Input: part model. Units: mm. Frame: model coordinates. A direction names the side the tool comes from. Coordinates: 2 decimals unless noted, no trailing zeros. Write each loop counter-clockwise with the first axis right and the second up, starting at its lowest first coordinate (ties: lowest second). Pieces come first, ordered by that corner, then holes. Notation, with made-up numbers: M 53,-37.5 L 92,-37.5 A36 cw 92,-0.5 Z; hole C 46.25,86.5 d7. An arc over 180 degrees is marked long. Use one line per item in the form item = value.
from build123d import *

# Parameters (mm, degrees)
F0_W     = 200.66
F0_H     = 63.5
F1_DEPTH = 63.5
F2_W     = 200.66
F2_H     = 12.954
F2_W_2   = 175.26
F3_DEPTH = 3.1242


with BuildPart() as f1:
    # F0 (on Top) → F1 (new body)
    with BuildSketch(Plane.XY):
        with Locations((-100.33, 31.75)):
            Rectangle(F0_W, F0_H)
    extrude(amount=-F1_DEPTH)

    # F2 (on face) → F3 (cut)
    with BuildSketch(Plane.XY):
        with Locations((-100.33, 6.477)):
            Rectangle(F2_W, F2_H)
        with Locations((-87.63, 57.023)):
            Rectangle(F2_W_2, F2_H)
    extrude(amount=-F3_DEPTH, mode=Mode.SUBTRACT)


solid = f1.part
(1) Line query: probe 1 along Z at (x, y) = (-104, 57). Output: solid intervals per line, ascending.
Computed:
probe_1 = -63.5 to -3.12
(2) Section query B-B on y = 11. Return the cut outline in (x, z).
Computed:
outline = M -200.66,-63.5 L 0,-63.5 L 0,-3.12 L -200.66,-3.12 Z
(3) Set-up query: faces 1 (the flat face through (-89, 57, -3.124)), 2 (the flat face through (-102, 7, -3.124)), 3 (the flat face through (-102, 33, 0)). Return all of +Z, -Z, +X, -X, +Y, -Y with unobstructed straight access to the full face (end or side cutting, diameter ignored); none if empty.
Computed:
face_1 = +Z, +X, +Y
face_2 = +Z, +X, -X, -Y
face_3 = +Z, +X, -X, +Y, -Y
(4) First-contact query: pin 1 Ø4 at (x, y) = (-123.5, 55.5) entering from +Z; pin 2 Ø0.9 at (x, z) = (-128, -1) entering from +Y; pin 3 Ø0.9 at (x, z) = (-59.5, -1) entering from -Y. Flat tips, straight axial feed; report the tip coordinate or a pass-through.
Computed:
pin_1 = -3.12
pin_2 = 50.55
pin_3 = 12.95
(5) Section query A-A on x = -102. Return the cut outline in (y, z).
Computed:
outline = M 0,-63.5 L 63.5,-63.5 L 63.5,-3.12 L 50.55,-3.12 L 50.55,0 L 12.95,0 L 12.95,-3.12 L 0,-3.12 Z
